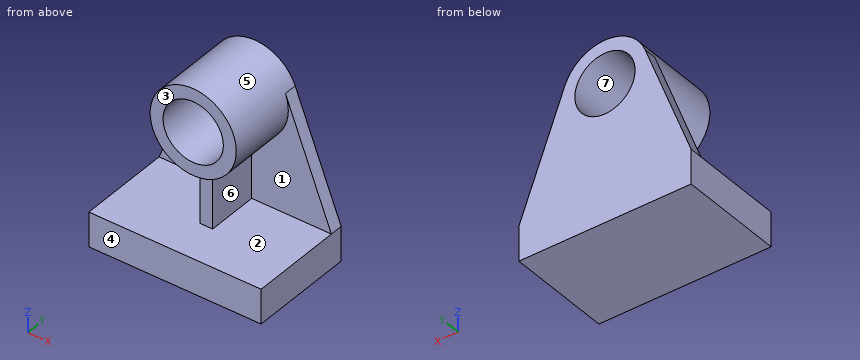
```python
from build123d import *

# Parameters (mm, degrees)
F0_R     = 44.45
F1_DEPTH = 19.05
F2_W     = 254
F2_H     = 50.8
F3_DEPTH = 137.16
F4_R     = 63.5
F4_R_2   = 44.45
F5_DEPTH = 101.6
F6_W     = 19.05
F6_H     = 89.6184392118
F7_DEPTH = 76.2


with BuildPart() as f1:
    # F0 (on Front) → F1 (new body)
    with BuildSketch(Plane.XZ):
        with BuildLine():
            ThreePointArc((-59.2277468166, 22.8981223472), (-11.6466320699, -62.4228000127), (63.5, 0))
            ThreePointArc((63.5, 0), (62.4228000127, 11.6466320699), (59.2277468166, 22.8981223472))
            ThreePointArc((59.2277468166, 22.8981223472), (0, 63.5), (-59.2277468166, 22.8981223472))
        make_face()
        Circle(F0_R, mode=Mode.SUBTRACT)
        with BuildLine():
            ThreePointArc((59.2277468166, 22.8981223472), (62.4228000127, 11.6466320699), (63.5, 0))
            ThreePointArc((63.5, 0), (-11.6466320699, -62.4228000127), (-59.2277468166, 22.8981223472))
            Line((-59.2277468166, 22.8981223472), (-127, -152.4))
            Line((-127, -152.4), (-127, -203.2))
            Line((-127, -203.2), (127, -203.2))
            Line((127, -203.2), (127, -152.4))
            Line((127, -152.4), (59.2277468166, 22.8981223472))
        make_face()
    extrude(amount=F1_DEPTH)

    # F2 (on face) → F3 (join)
    with BuildSketch(Plane.XZ.offset(19.05)):
        with Locations((0, -177.8)):
            Rectangle(F2_W, F2_H)
    extrude(amount=F3_DEPTH)

    # F4 (on face) → F5 (join)
    with BuildSketch(Plane.XZ.offset(19.05)):
        Circle(F4_R)
        Circle(F4_R_2, mode=Mode.SUBTRACT)
    extrude(amount=F5_DEPTH)

    # F6 (on face) → F7 (join)
    with BuildSketch(Plane.XZ.offset(19.05)):
        with Locations((0, -107.5907803941)):
            Rectangle(F6_W, F6_H)
    extrude(amount=F7_DEPTH)


solid = f1.part
```
Work out the finished part from the listing and answer in its coordinate system (mm). Face numbers are marked on the shaded views. A direction names the side the tool comes from. Give positions to 0.01 mm unless a question says otherwise; leave off trailing zeros. Loops run counter-clockwise (first coordinate to the right, second up) from the corner with the lowest first, then second, coordinate; pieces in that order, holes last. Notation, with made-up numbers: (88, 45) -> (97, 45) arc R19 ccw to (97, 66) -> close; hole circle Ø5 at (19, 25.25). An arc over 180 degrees is marked (long way). Put each result on its own line as item: value. Start each with the question number.
Item 1: Which of the six approach directions +Z, -Z, +X, -X, +Y, -Y give full straight-line access (tool end or side, diameter ignored) to the marked faces 1, 2 and 3?
Item 2: The part is cut by section D-D (y = -49). Give the vertices of the cut face in (x, z) (3 decimals), then the cut area to 3 significant figures.
Item 3: The mould has two halves that part along X. Classify the marked faces 4, 5, 6 and 7: released by +X, released by -X, zero draft, split by the parting line, or undercut.
Item 4: The part is cut by section A-A (y = -115.5). Give the vertices of the cut face in (x, z), then the cut area to 3 significant figures.
Item 5: The part is cut by section C-C (x = 0). Give the vertices of the cut face in (y, z), then the cut area to 3 significant figures.
Item 6: The part is cut by section B-B (z = 0). Give the vertices of the cut face in (x, y).
Item 7: Each of these flat-tipped pins is pushed along its axis until it touches: P1, Ø8, axis at x = 70, y = -96.5, coming from the +Z side; P2, Ø10, axis at x = 47.5, z = -92.5, coming from the -Y side; P3, Ø21, axis at x = 4.5, z = -112.5, coming from the -Y side; P4, Ø5, axis at x = 38.5, z = -65.5, coming from the +Y side. Where does it stop, or does it pass through?
Item 8: Find the intervals of material crossed by L1, parallel to Z at x = 0, y = -40.5; L2, parallel to Z at x = -107, y = -64.5; L3, parallel to Y at x = -3, z = 51, in increasing order. Write a range as [from, to].
Answers below:
1. face 1: +X, -Y
1. face 2: -Y
1. face 3: +Z, +X, -X, -Y
2. outline: (-127, -203.2) -> (127, -203.2) -> (127, -152.4) -> (9.525, -152.4) -> (9.525, -62.782) arc R63.5 ccw (long way) to (-9.525, -62.782) -> (-9.525, -152.4) -> (-127, -152.4) -> close; hole circle Ø88.9 at (0, 0)
2. area: 21,100 mm2
3. face 4: zero draft
3. face 5: split by the parting line
3. face 6: released by +X
3. face 7: undercut
4. outline: (-127, -203.2) -> (127, -203.2) -> (127, -152.4) -> (-127, -152.4) -> close; circle Ø127 at (0, 0); hole circle Ø88.9 at (0, 0)
4. area: 19,400 mm2
5. outline: (-156.21, -203.2) -> (0, -203.2) -> (0, -44.45) -> (-120.65, -44.45) -> (-120.65, -63.5) -> (-95.25, -63.5) -> (-95.25, -152.4) -> (-156.21, -152.4) -> close; (-120.65, 44.45) -> (0, 44.45) -> (0, 63.5) -> (-120.65, 63.5) -> close
5. area: 21,000 mm2
6. outline: (-68.08, -19.05) -> (-63.5, -19.05) -> (-63.5, -120.65) -> (-44.45, -120.65) -> (-44.45, 0) -> (-68.08, 0) -> close; (44.45, -120.65) -> (63.5, -120.65) -> (63.5, -19.05) -> (68.08, -19.05) -> (68.08, 0) -> (44.45, 0) -> close
7. P1: z = -152.4
7. P2: y = -19.05
7. P3: y = -95.25
7. P4: y = 0
8. L1: [-203.2, -44.45], [44.45, 63.5]
8. L2: [-203.2, -152.4]
8. L3: [-120.65, 0]
